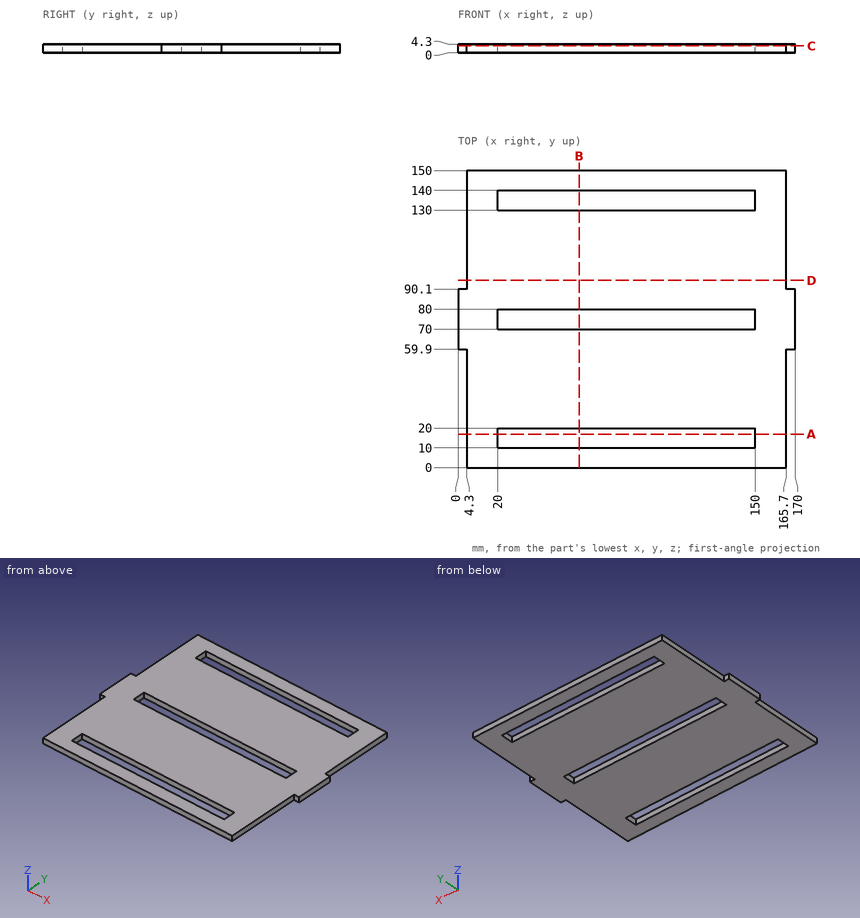
Could you check a few things on this drawing? It's one solid part, dimensions in mm from its lowest x, y, z. Coordinates: 2 decimals unless noted, no trailing zeros. Loops run counter-clockwise (first coordinate to the right, second up) from the corner with the lowest first, then second, coordinate; pieces in that order, holes last.
1. For P1, Ø2, axis at x = 62.5, z = 3, coming from the -Y side; P2, Ø2, axis at y = 117.5, z = 2.5, coming from the -X side; P3, Ø1.5, axis at y = 134, z = 0.5, coming from the +X side, each with a flat end and sliding along its axis, tell me the tip position at first contact or that it passes through.
2. Imagine slicing it at D-D (y = 94.5). Please give me the cut outline in (x, z).
3. Imagine slicing it at B-B (x = 61). Please give me the cut outline in (y, z).
4. I need wall thicknesses on L1, parallel to Y at x = 113, z = 1.55; L2, parallel to X at y = 71, z = 1.75; L3, parallel to X at y = 144, z = 2.1. Which ranges of each line are inside material? Lowest first, please.
5. Imagine slicing it at C-C (z = 3.4). Please give me the cut outline in (x, y), and give its area (3 significant figures).
6. Imagine slicing it at A-A (y = 17). Please give me the cut outline in (x, z), and give its area (3 significant figures).
Computed values:
1. P1: stops at y = 0
1. P2: stops at x = 4.3
1. P3: stops at x = 165.7
2. outline: (4.3, 0) - (165.7, 0) - (165.7, 4.3) - (4.3, 4.3) - close
3. outline: (0, 0) - (10, 0) - (10, 4.3) - (0, 4.3) - close; (20, 0) - (70, 0) - (70, 4.3) - (20, 4.3) - close; (80, 0) - (130, 0) - (130, 4.3) - (80, 4.3) - close; (140, 0) - (150, 0) - (150, 4.3) - (140, 4.3) - close
4. L1: y = 0 to 10, 20 to 70, 80 to 130, 140 to 150
4. L2: x = 0 to 20, 150 to 170
4. L3: x = 4.3 to 165.7
5. outline: (0, 59.9) - (4.3, 59.9) - (4.3, 0) - (165.7, 0) - (165.7, 59.9) - (170, 59.9) - (170, 90.1) - (165.7, 90.1) - (165.7, 150) - (4.3, 150) - (4.3, 90.1) - (0, 90.1) - close; hole (20, 10) - (150, 10) - (150, 20) - (20, 20) - close; hole (20, 70) - (150, 70) - (150, 80) - (20, 80) - close; hole (20, 130) - (150, 130) - (150, 140) - (20, 140) - close
5. area: 20,600 mm2
6. outline: (4.3, 0) - (20, 0) - (20, 4.3) - (4.3, 4.3) - close; (150, 0) - (165.7, 0) - (165.7, 4.3) - (150, 4.3) - close
6. area: 135 mm2
